Can you work these out from the drawing? Everything is in mm from the part's minimum corner. A direction names the side the tool comes from. Give positions to 0.01 mm unless a question says otherwise; leave off trailing zeros. Loops run counter-clockwise (first coordinate to the right, second up) from the corner with the lowest first, then second, coordinate; pieces in that order, holes last. Notation, with made-up numbers: M 42,-35.5 L 92,-35.5 A23 cw 92,-5.5 Z; hole C 11.25,-26.75 d5. An arc over 180 degrees is marked long. Use CSV: the item, a comma, the result in double quotes.
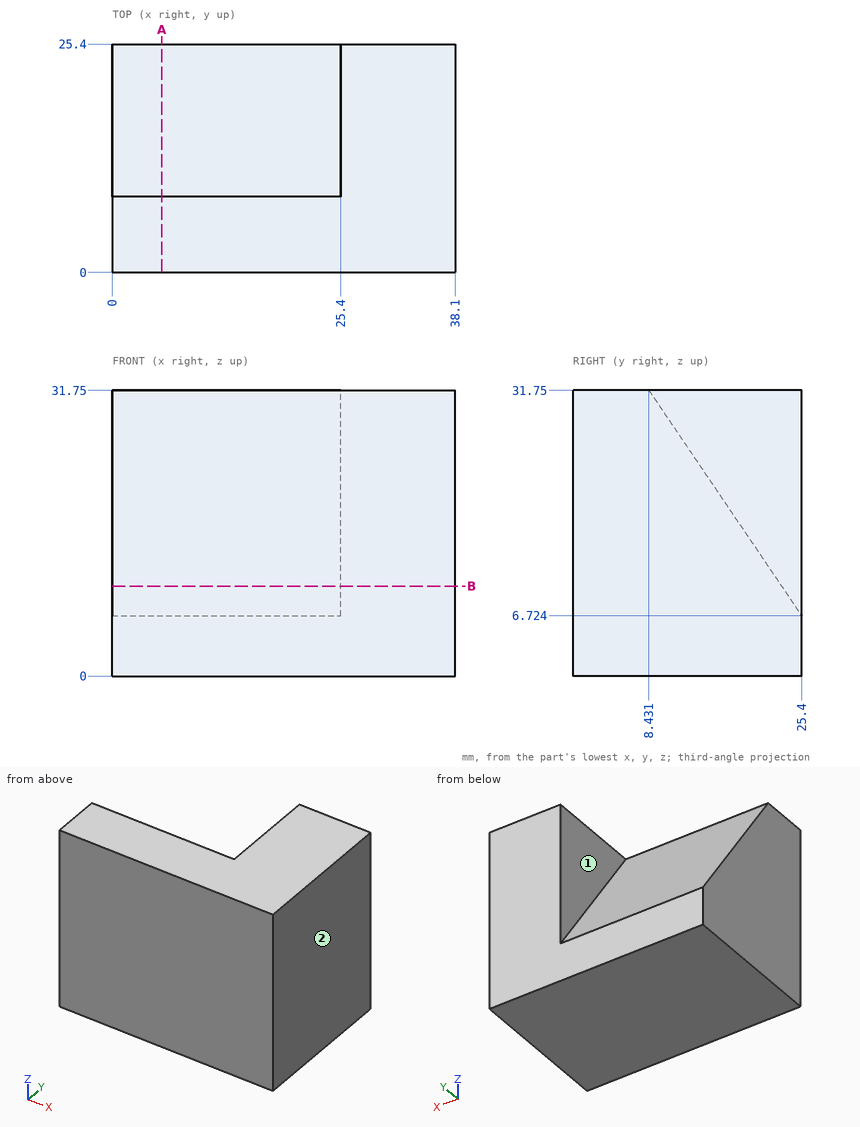
Q1. I want a section at B-B, the plane z = 10. Please give me the cut outline in (x, y), then the cut area to 3 significant figures.
Model answer:
outline,"M 0,0 L 38.1,0 L 38.1,25.4 L 25.4,25.4 L 25.4,23.18 L 0,23.18 Z"
area,"911 mm2"
Q2. I'm going to push flat-ended pins straight in: P1, Ø10, axis at y = 9.5, z = 5.5, coming from the -X side; P2, Ø4, axis at x = 17.5, z = 15, coming from the +Y side (1 decimal); P3, Ø3, axis at x = 14, z = 10.5, coming from the +Y side. Where does each tip first touch, or does it pass through?
Model answer:
P1,"x = 0"
P2,"y = 21.1"
P3,"y = 23.86"
Q3. I want a section at A-A, the plane x = 5.5. Please give me the cut outline in (y, z).
Model answer:
outline,"M 0,0 L 25.4,0 L 25.4,6.72 L 8.43,31.75 L 0,31.75 Z"
Q4. For the marked faces 1 and 2, which set-ups out of +Z, -Z, +X, -X, +Y, -Y let a thin tool reach every point of the face, with its end or its side?
Model answer:
face 1,"+Z, -X, +Y"
face 2,"+Z, -Z, +X, +Y, -Y"
Q5. Please list where these lines run through material, in increasing order: L1, parallel to X at y = 23.25, z = 25; L2, parallel to Y at x = 19, z = 13 (1 decimal); L3, parallel to Z at x = 8, y = 15.75 (1 decimal). Write a range as from..to.
Model answer:
L1,"25.4..38.1"
L2,"0..21.1"
L3,"0..21"
